from build123d import *

# Parameters (mm, degrees)
F0_W      = 15.55
F0_H      = 12.85
F1_DEPTH  = 7.86
F2_R      = 2.445
F3_DEPTH  = 5.74
F4_R      = 1.99
F5_DEPTH  = 25
F7_DEPTH  = 25
F8_R      = 0.314277
F8_R_2    = 0.345703
F9_DEPTH  = 0.2
F8_W      = 0.334352
F8_H      = 12.85
F10_DEPTH = 0.2
F12_DEPTH = 0.1
F13_W     = 2.232052
F13_H     = 0.354293
F14_DEPTH = 0.18
F15_DEPTH = 0.2


with BuildPart() as f1:
    # F0 (on Front) → F1 (new body)
    with BuildSketch(Plane.XZ):
        with Locations((-41.583441, 38.916974)):
            Rectangle(F0_W, F0_H)
    extrude(amount=F1_DEPTH)

    # F2 (on face) → F3 (join)
    with BuildSketch(Plane.XY.offset(45.341974)):
        with Locations((-41.583441, -3.93)):
            Circle(F2_R)
    extrude(amount=F3_DEPTH)

    # F4 (on face) → F5 (cut)
    with BuildSketch(Plane.YZ.offset(-33.808441)):
        with Locations((-3.93, 41.181974)):
            Circle(F4_R)
    extrude(amount=-F5_DEPTH, mode=Mode.SUBTRACT)

    # F6 (on face) → F7 (cut)
    with BuildSketch(Plane.XZ.offset(7.86)):
        Polygon((-49.358441, 45.341974), (-49.358441, 32.491974), (-47.458441, 45.341974), align=None)
        Polygon((-35.708441, 45.341974), (-33.808441, 32.491974), (-33.808441, 45.341974), align=None)
    extrude(amount=-F7_DEPTH, mode=Mode.SUBTRACT)

    # F8 (on face) → F9 (cut)
    with BuildSketch(Plane.XZ.offset(7.86)):
        with Locations((-40.971532, 39.419685)):
            Circle(F8_R)
        with Locations((-40.940102, 42.593867)):
            Circle(F8_R_2)
        with Locations((-40.877249, 35.554096)):
            Circle(F8_R_2)
    extrude(amount=-F9_DEPTH, mode=Mode.SUBTRACT)

    # F8 (on face) → F10 (cut)
    with BuildSketch(Plane.XZ.offset(7.86)):
        with Locations((-40.940102, 42.593867)):
            Circle(F8_R_2)
        with Locations((-40.971532, 39.419685)):
            Circle(F8_R)
        with Locations((-40.877249, 35.554096)):
            Circle(F8_R_2)
        with Locations((-41.750617, 38.916974)):
            Rectangle(F8_W, F8_H)
    extrude(amount=-F10_DEPTH, mode=Mode.SUBTRACT)

    # F11 (on face) → F12 (join)
    with BuildSketch(Plane.XZ.offset(7.86)):
        Polygon((-42.515382, 43.422379), (-41.917793, 43.885078), (-44.012314, 45.341974), align=None)
        Polygon((-39.660979, 45.341974), (-41.529234, 43.885078), (-40.948099, 43.422379), align=None)
    extrude(amount=F12_DEPTH)

    # F13 (on face) → F14 (join)
    with BuildSketch(Plane.XZ.offset(7.86)):
        with Locations((-44.771414, 42.786905)):
            Rectangle(F13_W, F13_H)
    extrude(amount=F14_DEPTH)

    # F13 (on face) → F15 (cut)
    with BuildSketch(Plane.XZ.offset(7.86)):
        with BuildLine():
            Line((-43.655388, 42.609759), (-45.88744, 42.609759))
            Line((-45.88744, 42.609759), (-45.88744, 40.218275))
            ThreePointArc((-45.88744, 40.218275), (-44.771414, 39.590548), (-43.655388, 40.218275))
            Line((-43.655388, 40.218275), (-43.655388, 42.609759))
        make_face()
    extrude(amount=-F15_DEPTH, mode=Mode.SUBTRACT)


solid = f1.part
The listing builds one solid part. Answer for the finished solid, in the listing's coordinates (mm). A direction names the side the tool comes from. Round coordinates to 2 decimals unless told otherwise and drop trailing zeros. Loops run counter-clockwise (first coordinate to the right, second up) from the corner with the lowest first, then second, coordinate; pieces in that order, holes last. Notation, with made-up numbers: M 33,88 L 61,88 A23 cw 61,106 Z; hole C -33,9.5 d9. An arc over 180 degrees is marked long. Write each question's results on one line, items separated by ' | '. Start each with the question number.
1) Find section D-D on y = -2.5. Write down the section's boundary in (x, z).
2) Each of these flat-tipped pins is pushed along its axis until it touches: pin 1 (2 mm diameter, centred on y = -2, z = 47.5, fed in from +X); pin 2 (2 mm diameter, centred on x = -42.5, z = 45, fed in from -Y); pin 3 (3 mm diameter, centred on x = -44.5, z = 48, fed in from -Y); pin 4 (4 mm diameter, centred on y = -2, z = 34.5, fed in from -X). Where does it stop, or does it pass through?
3) Determine the mould class of faces 6 (the flat face through (-42, -4, 32.492)), 7 (the cylindrical face through (-41.488, -4.189, 43.155)), 8 (the flat face through (-41, -7.96, 44)), 9 (the flat face through (-42, -4, 51.082)) for opening direction Z: pulls with the +Z half, pulls with the -Z half, needs draft (parallel to the pull), parting line crosses it, or undercut.
4) Find section C-C on z = 48.5. Write down the section's boundary in (x, y) (3 decimals).
5) Find section B-B on x = -43. Write down the section's boundary in (y, z).
6) Find section A-A on y = -3.93. Write down the section's boundary in (x, z).
7) Straight lines are drawn through the part: probe 1 along Z at (x, y) = (-38, -0.75); probe 2 along Y at (x, z) = (-36.75, 37.5); probe 3 along Z at (x, y) = (-43, -5.5). For each, find the intervals that lie inside material, in ascending order.
8) Which of the six approach directions +Z, -Z, +X, -X, +Y, -Y give full straight-line access (tool end or side, diameter ignored) to faces 1 (the flat face through (-48.42, -3.99, 38.83)), 2 (the flat face through (-43, -7.86, 45)), 3 (the flat face through (-45, -7.66, 41)), 4 (the cylindrical face through (-44.026, -3.822, 48.172)), 5 (the flat face through (-34.772, -3.985, 39.007))?
Final values:
1) outline: M -49.36,32.49 L -33.81,32.49 L -34.89,39.8 L -48.28,39.8 Z; M -47.87,42.57 L -35.3,42.57 L -35.71,45.34 L -39.6,45.34 L -39.6,51.08 L -43.57,51.08 L -43.57,45.34 L -47.46,45.34 Z
2) pin 1: x = -39.32 | pin 2: y = -7.96 | pin 3: y = -5.92 | pin 4: x = -49.36
3) face 6: pulls with the -Z half | face 7: undercut | face 8: needs draft | face 9: pulls with the +Z half
4) outline: C -41.583,-3.93 d4.89
5) outline: M -7.96,44.04 L -7.86,44.04 L -7.86,32.49 L 0,32.49 L 0,45.34 L -1.94,45.34 L -1.94,51.08 L -5.92,51.08 L -5.92,45.34 L -7.86,45.34 L -7.86,44.64 L -7.96,44.64 Z; hole C -3.93,41.18 d3.98
6) outline: M -49.36,32.49 L -33.81,32.49 L -34.8,39.19 L -48.37,39.19 Z; M -47.78,43.17 L -35.39,43.17 L -35.71,45.34 L -39.14,45.34 L -39.14,51.08 L -44.03,51.08 L -44.03,45.34 L -47.46,45.34 Z
7) probe 1: 32.49 to 45.34 | probe 2: -7.86 to 0 | probe 3: 32.49 to 39.96, 42.4 to 51.08
8) face 1: +Z, -X, +Y, -Y | face 2: +Z, -Y | face 3: -Y | face 4: +Z | face 5: +Z, +X, +Y, -Y
